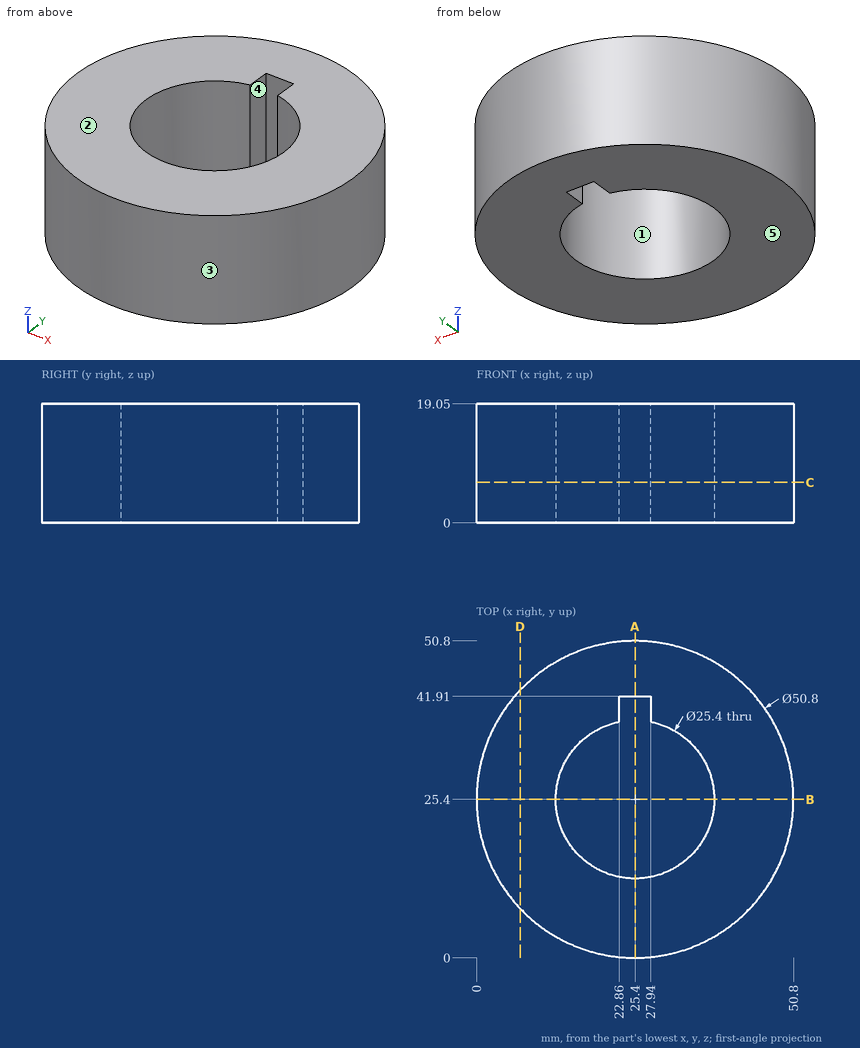
Geometry check sheet. Reference: drawing and pictorial views, mm from the part's lowest x, y, z. A direction names the side the tool comes from. Round coordinates to 2 decimals unless told otherwise and drop trailing zeros. Loops run counter-clockwise (first coordinate to the right, second up) from the corner with the lowest first, then second, coordinate; pieces in that order, holes last. Notation, with made-up numbers: M -36,36 L -21,36 A10 cw -21,55 Z; hole C 45.25,79 d5. An arc over 180 degrees is marked long. Return JSON: item names as keys, results as strings. Group by question number.
(1) Section check B-B, the plane y = 25.4. Enter the section's corners in (x, z).
(2) Mould release check, pull along Y, two halves, no side actions. Record for the marked faces 1, 2 and 3: pulls with the +Y half, pulls with the -Y half, needs draft (parallel to the pull), parting line crosses it, or undercut.
(3) Set-up check for the marked faces 4 and 5: record each of +Z, -Z, +X, -X, +Y, -Y from which the full face is reachable in a straight line by a thin tool's end or side.
(4) Scan lines: line 1 along Y through (x, z) = (25.4, 13); line 2 along X through (y, z) = (26, 13.75); line 3 along Y through (x, z) = (31.5, 8.5). Record each from-to range of solid material in increasing order. Write a range as [from, to].
(5) Section check D-D, the plane x = 7. Enter the section's corners in (y, z), and give its area (3 significant figures).
(6) Go/stop test with flat-tipped pins: pin 1 (4 mm diameter, centred on y = 40.5, z = 5.5, fed in from +X); pin 2 (4 mm diameter, centred on x = 22, z = 11, fed in from -Y); pin 3 (2 mm diameter, centred on x = 30, z = 5.5, fed in from +Y). Record where each tip stops, or that it passes through.
(7) Section check A-A, the plane x = 25.4. Enter the section's corners in (y, z), and give its area (3 significant figures).
(8) Section check C-C, the plane z = 6.5. Enter the section's corners in (x, y).
Data:
{
 "1": {"outline": "M 0,0 L 12.7,0 L 12.7,19.05 L 0,19.05 Z; M 38.1,0 L 50.8,0 L 50.8,19.05 L 38.1,19.05 Z"},
 "2": {"face 1": "undercut", "face 2": "needs draft", "face 3": "parting line crosses it"},
 "3": {"face 4": "+Z, -Z", "face 5": "-Z, +X, -X, +Y, -Y"},
 "4": {"line 1": "[0, 12.7], [41.91, 50.8]", "line 2": "[0.01, 12.71], [38.09, 50.79]", "line 3": "[0.74, 14.26], [36.54, 50.06]"},
 "5": {"outline": "M 7.89,0 L 42.91,0 L 42.91,19.05 L 7.89,19.05 Z", "area": "667 mm²"},
 "6": {"pin 1": "x = 47.16", "pin 2": "y = 0.04", "pin 3": "y = 50.54"},
 "7": {"outline": "M 0,0 L 12.7,0 L 12.7,19.05 L 0,19.05 Z; M 41.91,0 L 50.8,0 L 50.8,19.05 L 41.91,19.05 Z", "area": "411 mm²"},
 "8": {"outline": "C 25.4,25.4 d50.8; hole M 22.86,37.84 A12.7 ccw long 27.94,37.84 L 27.94,41.91 L 22.86,41.91 Z"}
}
